```python
from build123d import *

# Parameters (mm, degrees)
F1_DEPTH = 31.75
F2_W     = 19.05
F2_H     = 19.05
F3_DEPTH = 19.05
F5_DEPTH = 12.7
F7_DEPTH = 19.05


with BuildPart() as f1:
    # F0 (on Front) → F1 (new body)
    with BuildSketch(Plane.XZ):
        Polygon((-59.386093, 12.7), (-59.519075, 0), (-8.719075, 0), (-8.719075, 12.7), align=None)
        Polygon((-59.386093, 31.75), (-59.386093, 12.7), (-8.719075, 12.7), (-21.288181, 31.351074), align=None)
    extrude(amount=F1_DEPTH)

    # F2 (on face) → F3 (cut)
    with BuildSketch(Plane(origin=(-59.386093, 0, 0), x_dir=(0, -1, 0), z_dir=(-1, 0, 0))):
        with Locations((22.225, 22.225)):
            Rectangle(F2_W, F2_H)
    extrude(amount=-F3_DEPTH, mode=Mode.SUBTRACT)

    # F4 (on face) → F5 (cut)
    with BuildSketch(Plane(origin=(-40.336093, 0, 0), x_dir=(0, -1, 0), z_dir=(-1, 0, 0))):
        Polygon((12.7, 31.550526), (31.75, 12.7), (31.75, 31.550526), align=None)
    extrude(amount=-F5_DEPTH, mode=Mode.SUBTRACT)

    # F6 (on face) → F7 (cut)
    with BuildSketch(Plane.XZ.offset(31.75)):
        Polygon((-27.636093, 31.417544), (-27.636093, 12.7), (-8.719075, 12.7), (-21.288181, 31.351074), align=None)
    extrude(amount=-F7_DEPTH, mode=Mode.SUBTRACT)


solid = f1.part
```
Model file for the job. Use its own axes, mm. A direction names the side the tool comes from. Coordinates: 2 decimals unless noted, no trailing zeros. Write each loop counter-clockwise with the first axis right and the second up, starting at its lowest first coordinate (ties: lowest second). Pieces come first, ordered by that corner, then holes. Notation, with made-up numbers: (24.25, -27) - (61.25, -27) arc R23 cw to (61.25, -14) - close; hole circle Ø10 at (-27, -17). An arc over 180 degrees is marked (long way). One line per question, with ' | ' between items. Start each with the question number.
Q1. Cut at C-C, the plane x = -56. List the corners of the cut face in (y, z).
Q2. Cut at A-A, the plane y = -3. List the corners of the cut face in (x, z).
Q3. Cut at D-D, the plane z = 17.5. List the corners of the cut face in (x, y).
Q4. 3-axis set-ups, long thin cutter, end or side, ignore diameter. For faces 1 (the face through (-34, -31.75, 6)), 2 (the face through (-50, -22, 12.7)), 3 (the face through (-59.386, -6, 22)), 4 (the face through (-18, -22, 12.7)): which of +Z, -Z, +X, -X, +Y, -Y reach the whole face in a straight line?
Q5. Cut at B-B, the plane z = 22.5. List the corners of the cut face in (x, y).
Q6. Pin check, flat tips, straight feed: pin 1 (9.5 mm diameter, centred on x = -22.5, z = 20.5, fed in from -Y); pin 2 (5.5 mm diameter, centred on x = -16, y = -21.5, fed in from +Z); pin 3 (14 mm diameter, centred on y = -5, z = 21.5, fed in from -X). Stop position of each tip, or through.
Q7. Drill centre lines: line 1 (Z direction, x = -25.5, y = -13); line 2 (Y direction, x = -48, z = 13.5); line 3 (X direction, y = -18.5, z = 19). Where is each one in solid material? Low to high. Write a range as [from, to].
Answer below:
1) outline: (-31.75, 0) - (0, 0) - (0, 31.71) - (-12.7, 31.71) - (-12.7, 12.7) - (-31.75, 12.7) - close
2) outline: (-59.52, 0) - (-8.72, 0) - (-8.72, 12.7) - (-21.29, 31.35) - (-59.39, 31.75) - (-59.39, 12.7) - close
3) outline: (-59.39, -12.7) - (-40.34, -12.7) - (-40.34, -26.9) - (-27.64, -26.9) - (-27.64, -12.7) - (-11.95, -12.7) - (-11.95, 0) - (-59.39, 0) - close
4) face 1: +Z, -Z, +X, -X, -Y | face 2: +Z, -X, -Y | face 3: +Z, -X, +Y, -Y | face 4: +Z, +X, -Y
5) outline: (-59.39, -12.7) - (-40.34, -12.7) - (-40.34, -21.85) - (-27.64, -21.85) - (-27.64, -12.7) - (-15.32, -12.7) - (-15.32, 0) - (-59.39, 0) - close
6) pin 1: y = -12.7 | pin 2: z = 12.7 | pin 3: x = -59.39
7) line 1: [0, 12.7] | line 2: [-12.7, 0] | line 3: [-40.34, -27.64]
